from build123d import *

# Parameters (mm, degrees)
F0_W     = 1050.925
F0_H     = 1997.075
F1_DEPTH = 28.575
F2_W     = 993.775
F2_H     = 1939.925
F3_DEPTH = 82.55
F4_W     = 69.85
F4_H     = 69.85
F5_DEPTH = 647.7


with BuildPart() as f1:
    # F0 (on Top) → F1 (new body)
    with BuildSketch(Plane.XY):
        with Locations((1.311136, 625.877863)):
            Rectangle(F0_W, F0_H)
    extrude(amount=F1_DEPTH)

    # F2 (on face) → F3 (join)
    with BuildSketch(Plane.XY.offset(28.575)):
        with Locations((1.311136, 625.877863)):
            Rectangle(F2_W, F2_H)
    extrude(amount=F3_DEPTH)

    # F4 (on face) → F5 (join)
    with BuildSketch(Plane.XY.offset(111.125)):
        with Locations((-460.651364, 1560.915363)):
            Rectangle(F4_W, F4_H)
        with Locations((463.273636, 1560.915363)):
            Rectangle(F4_W, F4_H)
        with Locations((463.273636, -309.159637)):
            Rectangle(F4_W, F4_H)
        with Locations((-460.651364, -309.159637)):
            Rectangle(F4_W, F4_H)
    extrude(amount=F5_DEPTH)


solid = f1.part
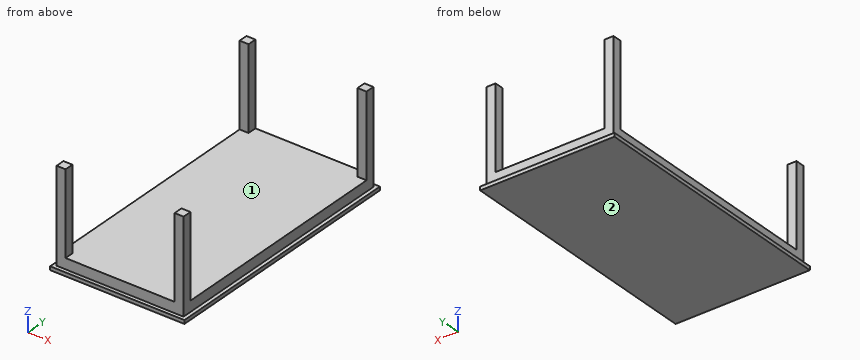
Geometry check sheet. Reference: the model listing, model coordinates, mm. Face numbers are marked on the shaded views. Coordinates: 2 decimals unless noted, no trailing zeros. Order: outer loops, then holes, each group sorted by start corner. A loop starts at its lowest first (then second) coordinate and runs counter-clockwise, first axis right, second up. Notation, with made-up numbers: (16.5, 26) - (22.5, 26) arc R11 cw to (22.5, 39) - close; hole circle Ø2 at (62.25, 72). An arc over 180 degrees is marked (long way). One line per item, written item: value.
(1) Sectioned sample at B-B (x = 227.5). Enter the section's corners in (y, z) (3 decimals).
Data:
outline: (-372.66, 0) - (1624.415, 0) - (1624.415, 28.575) - (1595.84, 28.575) - (1595.84, 111.125) - (-344.085, 111.125) - (-344.085, 28.575) - (-372.66, 28.575) - close
(2) Depth check by flat-ended pin: pin 1 Ø21 at (y, z) = (1570.5, 456.5) entering from +X; pin 2 Ø4 at (x, y) = (411, 535) entering from +Z (3 decimals); pin 3 Ø21 at (x, z) = (-462, 584) entering from -Y. Enter the tip coordinate at first touch or a pass-through.
Data:
pin 1: stops at x = 498.2
pin 2: stops at z = 111.125
pin 3: stops at y = -344.08
(3) Sectioned sample at D-D (z = 57.5). Enter the section's corners in (x, y).
Data:
outline: (-495.58, -344.08) - (498.2, -344.08) - (498.2, 1595.84) - (-495.58, 1595.84) - close
(4) Sectioned sample at C-C (y = -14.5). Enter the section's corners in (x, z) (3 decimals), and give its area (3 significant figures).
Data:
outline: (-524.151, 0) - (526.774, 0) - (526.774, 28.575) - (498.199, 28.575) - (498.199, 111.125) - (-495.576, 111.125) - (-495.576, 28.575) - (-524.151, 28.575) - close
area: 112,000 mm^2
(5) Sectioned sample at A-A (z = 206). Enter the section's corners in (x, y).
Data:
outline: (-495.58, -344.08) - (-425.73, -344.08) - (-425.73, -274.23) - (-495.58, -274.23) - close; (-495.58, 1525.99) - (-425.73, 1525.99) - (-425.73, 1595.84) - (-495.58, 1595.84) - close; (428.35, -344.08) - (498.2, -344.08) - (498.2, -274.23) - (428.35, -274.23) - close; (428.35, 1525.99) - (498.2, 1525.99) - (498.2, 1595.84) - (428.35, 1595.84) - close
(6) Release check for a two-part mould opening along Y. For the marked faces 1 and 2 record: +Y half, -Y half, draft (parallel to the pull), parting line (faces both ways), or undercut.
Data:
face 1: undercut
face 2: draft
(7) Thickness scan on probe 1 along Y at (x, z) = (456, 391); probe 2 along Z at (x, y) = (-426, -77.5) (3 decimals); probe 3 along X at (y, z) = (1307, 41). Record the ranges inside material, lowest first. Write a range as from..to.
Data:
probe 1: y = -344.08..-274.23, 1525.99..1595.84
probe 2: z = 0..111.125
probe 3: x = -495.58..498.2
